from build123d import *

# Parameters (mm, degrees)
BOSS_EXTRUDE1_DEPTH = 2
SKETCH3_W           = 5
SKETCH3_H           = 8
CUT_EXTRUDE1_DEPTH  = 2


with BuildPart() as part:
    # Sketch2 → Boss-Extrude1 (new body)
    with BuildSketch(Plane.XY):
        Polygon((-100.485199734, 17.220891199), (-80.485199734, 17.220891199), (-80.485199734, 14.220891199), (-70.485199734, 14.220891199), (-70.485199734, 6.220891199), (-80.485199734, 6.220891199), (-80.485199734, 3.220891199), (-100.485199734, 3.220891199), (-100.485199734, 6.220891199), (-103.485199734, 6.220891199), (-103.485199734, 14.220891199), (-100.485199734, 14.220891199), align=None)
        with BuildLine():
            Line((-90.485199734, 10.720891199), (-80.485199734, 10.720891199))
            ThreePointArc((-80.485199734, 10.720891199), (-79.485199734, 11.720891199), (-80.485199734, 12.720891199))
            Line((-80.485199734, 12.720891199), (-96.485199734, 12.720891199))
            ThreePointArc((-96.485199734, 12.720891199), (-97.485199734, 13.720891199), (-98.485199734, 12.720891199))
            Line((-98.485199734, 12.720891199), (-98.485199734, 6.220891199))
            ThreePointArc((-98.485199734, 6.220891199), (-97.485199734, 5.220891199), (-96.485199734, 6.220891199))
            Line((-96.485199734, 6.220891199), (-92.485199734, 6.220891199))
            ThreePointArc((-92.485199734, 6.220891199), (-91.485199734, 5.220891199), (-90.485199734, 6.220891199))
            Line((-90.485199734, 6.220891199), (-90.485199734, 10.720891199))
        make_face(mode=Mode.SUBTRACT)
    extrude(amount=BOSS_EXTRUDE1_DEPTH)

    # Sketch3 → Cut-Extrude1 (cut)
    with BuildSketch(Plane.XY.offset(2)):
        with Locations((-72.985199734, 10.220891199)):
            Rectangle(SKETCH3_W, SKETCH3_H)
    extrude(amount=-CUT_EXTRUDE1_DEPTH, mode=Mode.SUBTRACT)


solid = part.part
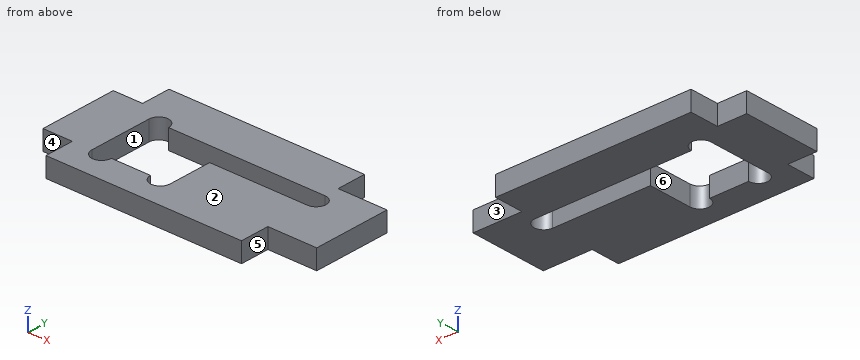
Source: CAD feature listing. Evaluate the final solid. Frame: model axes, mm. Face numbers are marked on the shaded views. A direction names the side the tool comes from. Coordinates: 2 decimals unless noted, no trailing zeros. Loops run counter-clockwise (first coordinate to the right, second up) from the corner with the lowest first, then second, coordinate; pieces in that order, holes last. Notation, with made-up numbers: (-7.75, -34.75) -> (20.25, -34.75) arc R21 ccw to (20.25, -29.75) -> close; hole circle Ø5 at (55, 57). An arc over 180 degrees is marked (long way). Answer in a Markdown table with one row per item. Add a question column.
Q1. Contact query for flat-ended pins moving along their axis: pin 1 Ø1 at (x, z) = (-102, 1.5) entering from +Y; pin 2 Ø4 at (x, y) = (-94.5, 10) entering from +Z; pin 3 Ø1 at (y, z) = (16, 1) entering from -X; pin 4 Ø0.6 at (y, z) = (5, 1) entering from +X. Output: stop coordinate, or through.
Q2. Section C-C on y = 12.25. Return the cut outline in (x, z).
Q3. Ray query, line 1 along Y through (x, z) = (-82.5, 1.25); line 2 along X through (y, z) = (10.25, 1.15); line 3 along Y through (x, z) = (-97.25, 1.8). Return the intervals inside material, ascending.
Q4. Section D-D on y = 4.75. Return the cut outline in (x, z).
Q5. Pull-direction query (Y, two-part tool) for the marked faces 1, 2 and 3; classes: pulls with the +Y half, pulls with the -Y half, needs draft (parallel to the pull), parting line crosses it, or undercut.
Q6. Section B-B on z = 0.3. Return the cut outline in (x, y), and give its area (3 significant figures).
Q7. Reachability of the marked faces 4, 5 and 6 from +Z, -Z, +X, -X, +Y, -Y: full face, straight path, thin tool, end or side. Return the list, or none.
Q8. Section A-A on x = -83.5. Return the cut outline in (y, z), and give its area (3 significant figures).
Computed values:
| question | item | result |
|---|---|---|
| 1 | pin 1 | stops at y = 14.22 |
| 1 | pin 2 | passes through |
| 1 | pin 3 | stops at x = -100.49 |
| 1 | pin 4 | stops at x = -80.49 |
| 2 | outline | (-103.49, 0) -> (-98.49, 0) -> (-98.49, 2) -> (-103.49, 2) -> close; (-79.64, 0) -> (-75.49, 0) -> (-75.49, 2) -> (-79.64, 2) -> close |
| 3 | line 1 | y = 3.22 to 10.72, 12.72 to 17.22 |
| 3 | line 2 | x = -103.49 to -98.49, -90.49 to -75.49 |
| 3 | line 3 | y = 3.22 to 5.25, 13.69 to 17.22 |
| 4 | outline | (-100.49, 0) -> (-80.49, 0) -> (-80.49, 2) -> (-100.49, 2) -> close |
| 5 | face 1 | undercut |
| 5 | face 2 | needs draft |
| 5 | face 3 | pulls with the +Y half |
| 6 | outline | (-103.49, 6.22) -> (-100.49, 6.22) -> (-100.49, 3.22) -> (-80.49, 3.22) -> (-80.49, 6.22) -> (-75.49, 6.22) -> (-75.49, 14.22) -> (-80.49, 14.22) -> (-80.49, 17.22) -> (-100.49, 17.22) -> (-100.49, 14.22) -> (-103.49, 14.22) -> close; hole (-98.49, 6.22) arc R1 ccw to (-96.49, 6.22) -> (-92.49, 6.22) arc R1 ccw to (-90.49, 6.22) -> (-90.49, 10.72) -> (-80.49, 10.72) arc R1 ccw to (-80.49, 12.72) -> (-96.49, 12.72) arc R1 ccw to (-98.49, 12.72) -> close |
| 6 | area | 266 mm^2 |
| 7 | face 4 | +Z, -Z, -X, -Y |
| 7 | face 5 | +Z, -Z, +X, -Y |
| 7 | face 6 | +Z, -Z |
| 8 | outline | (3.22, 0) -> (10.72, 0) -> (10.72, 2) -> (3.22, 2) -> close; (12.72, 0) -> (17.22, 0) -> (17.22, 2) -> (12.72, 2) -> close |
| 8 | area | 24.0 mm^2 |
